```python
from build123d import *

# Parameters (mm, degrees)
F0_R     = 1.5
F1_DEPTH = 2


# Not quite as in the source:
# - a feature names something its author has since deleted; it is built from what else it names


with BuildPart() as f1:
    # F0 (on Top) → F1 (new body)
    with BuildSketch(Plane.XY):
        with BuildLine():
            Line((-61.8704294452, 175.1948396463), (-53.8704294452, 175.1948396463))
            Line((-53.8704294452, 175.1948396463), (-53.8704294452, 185.547974161))
            ThreePointArc((-53.8704294452, 185.547974161), (-57.1946545112, 183.1877510697), (-58.3269518777, 187.1042581875))
            ThreePointArc((-58.3269518777, 187.1042581875), (-59.9354051762, 184.8644644288), (-61.3162125777, 182.4775901096))
            ThreePointArc((-61.3162125777, 182.4775901096), (-61.7299003867, 181.366665728), (-61.8704294452, 180.1895751756))
            Line((-61.8704294452, 180.1895751756), (-61.8704294452, 175.1948396463))
        make_face()
        with Locations((-58.3704294452, 179.1948396463)):
            Circle(F0_R, mode=Mode.SUBTRACT)
        with BuildLine():
            ThreePointArc((-58.3269518777, 187.1042581875), (-57.1946545112, 183.1877510697), (-53.8704294452, 185.547974161))
            ThreePointArc((-53.8704294452, 185.547974161), (-54.6026624922, 187.315741114), (-56.3704294452, 188.047974161))
            ThreePointArc((-56.3704294452, 188.047974161), (-57.4565440648, 187.7997190473), (-58.3269518777, 187.1042581875))
        make_face()
        with BuildLine():
            Line((-18.8704294452, 175.1948396463), (-10.8704294452, 175.1948396463))
            Line((-10.8704294452, 175.1948396463), (-10.8704294452, 180.1895751756))
            ThreePointArc((-10.8704294452, 180.1895751756), (-11.0109585037, 181.366665728), (-11.4246463127, 182.4775901096))
            ThreePointArc((-11.4246463127, 182.4775901096), (-12.8054541473, 184.8644650992), (-14.4139080064, 187.1042594368))
            ThreePointArc((-14.4139080064, 187.1042594368), (-14.010206617, 186.3721999805), (-13.8704294452, 185.547974161))
            ThreePointArc((-13.8704294452, 185.547974161), (-16.3704294452, 183.047974161), (-18.8704294452, 185.547974161))
            Line((-18.8704294452, 185.547974161), (-18.8704294452, 175.1948396463))
        make_face()
        with Locations((-14.3704294452, 179.1948396463)):
            Circle(F0_R, mode=Mode.SUBTRACT)
        with BuildLine():
            ThreePointArc((-16.3704294452, 188.047974161), (-18.1381963982, 187.315741114), (-18.8704294452, 185.547974161))
            ThreePointArc((-18.8704294452, 185.547974161), (-16.3704294452, 183.047974161), (-13.8704294452, 185.547974161))
            ThreePointArc((-13.8704294452, 185.547974161), (-14.010206617, 186.3721999805), (-14.4139080064, 187.1042594368))
            ThreePointArc((-14.4139080064, 187.1042594368), (-15.2843155445, 187.7997193941), (-16.3704294452, 188.047974161))
        make_face()
        with BuildLine():
            Line((-36.3704294452, 166.6948396463), (-36.3704294452, 165.1948396463))
            Line((-36.3704294452, 165.1948396463), (-23.8704294452, 165.1948396463))
            ThreePointArc((-23.8704294452, 165.1948396463), (-20.3348955393, 166.6593057403), (-18.8704294452, 170.1948396463))
            Line((-18.8704294452, 170.1948396463), (-18.8704294452, 175.1948396463))
            Line((-18.8704294452, 175.1948396463), (-34.8704294452, 175.1948396463))
            Line((-34.8704294452, 175.1948396463), (-34.8704294452, 168.1948396463))
            ThreePointArc((-34.8704294452, 168.1948396463), (-35.3097692734, 167.1341794745), (-36.3704294452, 166.6948396463))
        make_face()
        with BuildLine():
            Line((-48.8704294452, 165.1948396463), (-36.3704294452, 165.1948396463))
            Line((-36.3704294452, 165.1948396463), (-36.3704294452, 166.6948396463))
            ThreePointArc((-36.3704294452, 166.6948396463), (-37.431089617, 167.1341794745), (-37.8704294452, 168.1948396463))
            Line((-37.8704294452, 168.1948396463), (-37.8704294452, 175.1948396463))
            Line((-37.8704294452, 175.1948396463), (-53.8704294452, 175.1948396463))
            Line((-53.8704294452, 175.1948396463), (-53.8704294452, 170.1948396463))
            ThreePointArc((-53.8704294452, 170.1948396463), (-52.4059633511, 166.6593057403), (-48.8704294452, 165.1948396463))
        make_face()
        with BuildLine():
            Line((-34.8704294452, 175.1948396463), (-18.8704294452, 175.1948396463))
            Line((-18.8704294452, 175.1948396463), (-18.8704294452, 185.547974161))
            Line((-18.8704294452, 185.547974161), (-18.8704294452, 188.047974161))
            Line((-18.8704294452, 188.047974161), (-53.8704294452, 188.047974161))
            Line((-53.8704294452, 188.047974161), (-53.8704294452, 185.547974161))
            Line((-53.8704294452, 185.547974161), (-53.8704294452, 175.1948396463))
            Line((-53.8704294452, 175.1948396463), (-37.8704294452, 175.1948396463))
            ThreePointArc((-37.8704294452, 175.1948396463), (-36.3704294452, 176.6948396463), (-34.8704294452, 175.1948396463))
        make_face()
        with BuildLine():
            ThreePointArc((-41.6596574736, 160.2762349793), (-39.1836561071, 161.7003703018), (-36.3704294452, 162.1948396463))
            Line((-36.3704294452, 162.1948396463), (-36.3704294452, 165.1948396463))
            Line((-36.3704294452, 165.1948396463), (-48.8704294452, 165.1948396463))
            ThreePointArc((-48.8704294452, 165.1948396463), (-52.4059633511, 166.6593057403), (-53.8704294452, 170.1948396463))
            Line((-53.8704294452, 170.1948396463), (-53.8704294452, 175.1948396463))
            Line((-53.8704294452, 175.1948396463), (-61.8704294452, 175.1948396463))
            Line((-61.8704294452, 175.1948396463), (-61.8704294452, 161.6948396463))
            ThreePointArc((-61.8704294452, 161.6948396463), (-61.2846430076, 160.2806260839), (-59.8704294452, 159.6948396463))
            Line((-59.8704294452, 159.6948396463), (-43.2624538212, 159.6948396463))
            ThreePointArc((-43.2624538212, 159.6948396463), (-45.0302207742, 163.9626065992), (-40.7624538212, 162.1948396463))
            ThreePointArc((-40.7624538212, 162.1948396463), (-40.997835656, 161.13582852), (-41.6596574736, 160.2762349793))
        make_face()
        with Locations((-58.3704294452, 164.1948396463)):
            Circle(F0_R, mode=Mode.SUBTRACT)
        with BuildLine():
            ThreePointArc((-43.2624538212, 159.6948396463), (-42.4099609085, 159.8446788361), (-41.6596574736, 160.2762349793))
            ThreePointArc((-41.6596574736, 160.2762349793), (-40.997835656, 161.13582852), (-40.7624538212, 162.1948396463))
            ThreePointArc((-40.7624538212, 162.1948396463), (-45.0302207742, 163.9626065992), (-43.2624538212, 159.6948396463))
        make_face()
        with BuildLine():
            ThreePointArc((-56.3704294452, 188.047974161), (-54.6026624922, 187.315741114), (-53.8704294452, 185.547974161))
            Line((-53.8704294452, 185.547974161), (-53.8704294452, 188.047974161))
            Line((-53.8704294452, 188.047974161), (-56.3704294452, 188.047974161))
        make_face()
        with BuildLine():
            Line((-18.8704294452, 188.047974161), (-18.8704294452, 185.547974161))
            ThreePointArc((-18.8704294452, 185.547974161), (-18.1381963982, 187.315741114), (-16.3704294452, 188.047974161))
            Line((-16.3704294452, 188.047974161), (-18.8704294452, 188.047974161))
        make_face()
        with BuildLine():
            ThreePointArc((-26.9784050691, 162.1948396463), (-27.7106381162, 160.4270726933), (-29.4784050691, 159.6948396463))
            Line((-29.4784050691, 159.6948396463), (-12.8704294452, 159.6948396463))
            ThreePointArc((-12.8704294452, 159.6948396463), (-11.4562158828, 160.2806260839), (-10.8704294452, 161.6948396463))
            Line((-10.8704294452, 161.6948396463), (-10.8704294452, 175.1948396463))
            Line((-10.8704294452, 175.1948396463), (-18.8704294452, 175.1948396463))
            Line((-18.8704294452, 175.1948396463), (-18.8704294452, 170.1948396463))
            ThreePointArc((-18.8704294452, 170.1948396463), (-20.3348955393, 166.6593057403), (-23.8704294452, 165.1948396463))
            Line((-23.8704294452, 165.1948396463), (-36.3704294452, 165.1948396463))
            Line((-36.3704294452, 165.1948396463), (-36.3704294452, 162.1948396463))
            ThreePointArc((-36.3704294452, 162.1948396463), (-33.557202708, 161.7003702745), (-31.0812012938, 160.2762348766))
            ThreePointArc((-31.0812012938, 160.2762348766), (-30.5374162679, 164.4594577776), (-26.9784050691, 162.1948396463))
        make_face()
        with Locations((-14.3704294452, 164.1948396463)):
            Circle(F0_R, mode=Mode.SUBTRACT)
        with BuildLine():
            ThreePointArc((-31.0812012938, 160.2762348766), (-30.3308979066, 159.8446788088), (-29.4784050691, 159.6948396463))
            ThreePointArc((-29.4784050691, 159.6948396463), (-27.7106381162, 160.4270726933), (-26.9784050691, 162.1948396463))
            ThreePointArc((-26.9784050691, 162.1948396463), (-30.5374162679, 164.4594577776), (-31.0812012938, 160.2762348766))
        make_face()
        with BuildLine():
            Line((-53.8704294452, 188.047974161), (-18.8704294452, 188.047974161))
            Line((-18.8704294452, 188.047974161), (-18.8704294452, 191.5679000418))
            ThreePointArc((-18.8704294452, 191.5679000418), (-19.871628172, 192.3307748764), (-20.9060372255, 193.047974161))
            Line((-20.9060372255, 193.047974161), (-29.8583912725, 193.047974161))
            ThreePointArc((-29.8583912725, 193.047974161), (-36.3704294452, 189.6948396463), (-42.8824676178, 193.047974161))
            Line((-42.8824676178, 193.047974161), (-51.8348216648, 193.047974161))
            ThreePointArc((-51.8348216648, 193.047974161), (-52.8692307184, 192.3307748764), (-53.8704294452, 191.5679000418))
            Line((-53.8704294452, 191.5679000418), (-53.8704294452, 188.047974161))
        make_face()
        with BuildLine():
            Line((-56.3704294452, 188.047974161), (-53.8704294452, 188.047974161))
            Line((-53.8704294452, 188.047974161), (-53.8704294452, 191.5679000418))
            ThreePointArc((-53.8704294452, 191.5679000418), (-55.7861337119, 189.8913117759), (-57.5419746752, 188.047974161))
            Line((-57.5419746752, 188.047974161), (-56.3704294452, 188.047974161))
        make_face()
        with BuildLine():
            Line((-18.8704294452, 191.5679000418), (-18.8704294452, 188.047974161))
            Line((-18.8704294452, 188.047974161), (-16.3704294452, 188.047974161))
            Line((-16.3704294452, 188.047974161), (-15.1988842152, 188.047974161))
            ThreePointArc((-15.1988842152, 188.047974161), (-16.9547251785, 189.8913117759), (-18.8704294452, 191.5679000418))
        make_face()
        with BuildLine():
            ThreePointArc((-58.3269518777, 187.1042581875), (-57.4565440648, 187.7997190473), (-56.3704294452, 188.047974161))
            Line((-56.3704294452, 188.047974161), (-57.5419746752, 188.047974161))
            ThreePointArc((-57.5419746752, 188.047974161), (-57.939625189, 187.5804098217), (-58.3269518777, 187.1042581875))
        make_face()
        with BuildLine():
            Line((-15.1988842152, 188.047974161), (-16.3704294452, 188.047974161))
            ThreePointArc((-16.3704294452, 188.047974161), (-15.2843155445, 187.7997193941), (-14.4139080064, 187.1042594368))
            ThreePointArc((-14.4139080064, 187.1042594368), (-14.8012342118, 187.5804104353), (-15.1988842152, 188.047974161))
        make_face()
        with BuildLine():
            Line((-29.8583912725, 193.047974161), (-20.9060372255, 193.047974161))
            ThreePointArc((-20.9060372255, 193.047974161), (-23.799669125, 194.7209543402), (-26.8717251154, 196.0379358287))
            ThreePointArc((-26.8717251154, 196.0379358287), (-26.1524301853, 195.489141652), (-25.8795767704, 194.6265228146))
            ThreePointArc((-25.8795767704, 194.6265228146), (-27.6251244235, 193.1467571743), (-28.7991852371, 195.1109934548))
            ThreePointArc((-28.7991852371, 195.1109934548), (-29.2536378362, 194.0408996913), (-29.8583912725, 193.047974161))
        make_face()
        with BuildLine():
            ThreePointArc((-25.8795767704, 194.6265228146), (-26.1524301853, 195.489141652), (-26.8717251154, 196.0379358287))
            ThreePointArc((-26.8717251154, 196.0379358287), (-28.0296772719, 195.97832507), (-28.7991852371, 195.1109934548))
            ThreePointArc((-28.7991852371, 195.1109934548), (-27.6251244235, 193.1467571743), (-25.8795767704, 194.6265228146))
        make_face()
        with BuildLine():
            ThreePointArc((-43.9416738286, 195.1109939684), (-44.7111817722, 195.978325144), (-45.8691335854, 196.037935897))
            ThreePointArc((-45.8691335854, 196.037935897), (-46.2239010399, 193.3993762875), (-43.86128212, 194.6265228146))
            ThreePointArc((-43.86128212, 194.6265228146), (-43.8815165242, 194.8720707354), (-43.9416738286, 195.1109939684))
        make_face()
        with BuildLine():
            ThreePointArc((-45.8691335854, 196.037935897), (-48.9411896753, 194.7209543853), (-51.8348216648, 193.047974161))
            Line((-51.8348216648, 193.047974161), (-42.8824676178, 193.047974161))
            ThreePointArc((-42.8824676178, 193.047974161), (-43.4872211781, 194.0408999327), (-43.9416738286, 195.1109939684))
            ThreePointArc((-43.9416738286, 195.1109939684), (-43.8815165242, 194.8720707354), (-43.86128212, 194.6265228146))
            ThreePointArc((-43.86128212, 194.6265228146), (-46.2239010399, 193.3993762875), (-45.8691335854, 196.037935897))
        make_face()
    extrude(amount=F1_DEPTH)


solid = f1.part
```
Could you check a few things on this model? Use its own coordinates, in mm. A direction names the side the tool comes from. Coordinates: 2 decimals unless noted, no trailing zeros. Loops run counter-clockwise (first coordinate to the right, second up) from the corner with the lowest first, then second, coordinate; pieces in that order, holes last. Notation, with made-up numbers: M 52.5,81 L 104.5,81 A33 cw 104.5,119 Z; hole C -27.75,8 d6. An arc over 180 degrees is marked long. Put each result on its own line as item: value. Start each with the question number.
(1) Suppose I cut it at C-C on x = -32.5. Please give me the cut outline in (y, z).
(2) Suppose I cut it at B-B on y = 191. Please give me the cut outline in (x, z).
(3) I need wall thicknesses on line 1 (X direction, y = 163, z = 0.95); line 2 (Y direction, x = -57.5, z = 1.5); line 3 (X direction, y = 173, z = 1.5). Which ranges of each line are inside material? Lowest first, please. Write a range as from..to.
(4) Will this pin go through, and if not, where does the flat tip stop? P1, Ø5, axis at x = -14.37, y = 179.19, coming from the -Z side.
(5) Thinking about a two-plate mould opening in X: for faces 4 (the face through (-57.678, 162.864, 0.986)), 5 (the face through (-52, 159.695, 1)), 6 (the face through (-61.726, 181.383, 0.986)), which applies, pulls with the +X half, pulls with the -X half, needs draft (parallel to the pull), parting line crosses it, or undercut?
(6) Suppose I cut it at D-D on z = 0.75. Please give me the cut outline in (x, y).
(7) For faces 1 (the face through (-11.007, 181.35, 0.986)), 2 (the face through (-34.87, 172, 1)), 3 (the face through (-30.34, 159.85, 0.99)), which set-ups out of +Z, -Z, +X, -X, +Y, -Y let a thin tool reach every point of the face, with its end or its side?
(8) Suppose I cut it at A-A on y = 171. Please give me the cut outline in (x, z).
Solutions:
1. outline: M 161.23,0 L 190.69,0 L 190.69,2 L 161.23,2 Z
2. outline: M -54.56,0 L -40.75,0 L -40.75,2 L -54.56,2 Z; M -31.99,0 L -18.18,0 L -18.18,2 L -31.99,2 Z
3. line 1: x = -61.87..-59.28, -57.46..-15.28, -13.46..-10.87
3. line 2: y = 159.69..162.97, 165.42..177.97, 180.42..188.1
3. line 3: x = -61.87..-37.87, -34.87..-10.87
4. P1: stops at z = 0
5. face 4: undercut
5. face 5: needs draft
5. face 6: pulls with the -X half
6. outline: M -61.87,161.69 A2 ccw -59.87,159.69 L -43.26,159.69 A2.5 ccw -41.66,160.28 A8.25 cw -31.08,160.28 A2.5 ccw -29.48,159.69 L -12.87,159.69 A2 ccw -10.87,161.69 L -10.87,180.19 A5 ccw -11.42,182.48 A28.06 ccw -26.87,196.04 A1.5 ccw -28.8,195.11 A8 cw -43.94,195.11 A1.5 ccw -45.87,196.04 A28.06 ccw -61.32,182.48 A5 ccw -61.87,180.19 Z; hole C -58.37,164.19 d3; hole C -58.37,179.19 d3; hole M -37.87,168.19 A1.5 ccw -34.87,168.19 L -34.87,175.19 A1.5 ccw -37.87,175.19 Z; hole C -14.37,164.19 d3; hole C -14.37,179.19 d3
7. face 1: +Z, -Z, +X, +Y
7. face 2: +Z, -Z
7. face 3: +Z, -Z, -Y
8. outline: M -61.87,0 L -37.87,0 L -37.87,2 L -61.87,2 Z; M -34.87,0 L -10.87,0 L -10.87,2 L -34.87,2 Z
